Study the drawing (mm; zero at the part's minimum x, y, z) and answer. Coordinates: 2 decimals unless noted, no trailing zeros. Loops run counter-clockwise (first coordinate to the right, second up) from the corner with the lowest first, then second, coordinate; pieces in that order, holes last. Notation, with made-up numbers: (-25.75, 39.25) -> (19.25, 39.25) arc R35 ccw to (19.25, 75.25) -> close; hole circle Ø5 at (64.25, 20.5). An arc over 180 degrees is marked (long way). Answer as a JSON object with one key per item and string values. Group by question number.
Q1. Determine the mould class of the marked faces 1, 2 and 3 for opening direction Y: released by +Y, released by -Y, zero draft, split by the parting line, or undercut.
Q2. Straight lines are drawn through the part: line 1 along Y through (x, z) = (3, 50); line 2 along Y through (x, z) = (7.25, 50); line 3 along Y through (x, z) = (1, 49). For each, find the intervals that lie inside material, in ascending order. Write a range as [from, to].
Q3. The part is cut by section A-A on z = 50. Write down the section's boundary in (x, y), and give its area (3 significant figures).
Q4. Each of these flat-tipped pins is pushed along its axis until it touches: P1, Ø3, axis at x = 4, y = 142.5, coming from the +Z side; P2, Ø1.8, axis at y = 36, z = 49, coming from the -X side; P3, Ø5, axis at x = 7, y = 33.5, coming from the +Z side; P4, Ø9, axis at y = 180, z = 50, coming from the -X side. Where does it stop, or does it pass through?
Q5. The part is cut by section C-C on z = 78. Write down the section's boundary in (x, y), and give its area (3 significant figures).
Q6. The part is cut by section D-D on y = 35.5. Write down the section's boundary in (x, z), and give its area (3 significant figures).
Q7. The part is cut by section B-B on x = 7. Write down the section's boundary in (y, z).
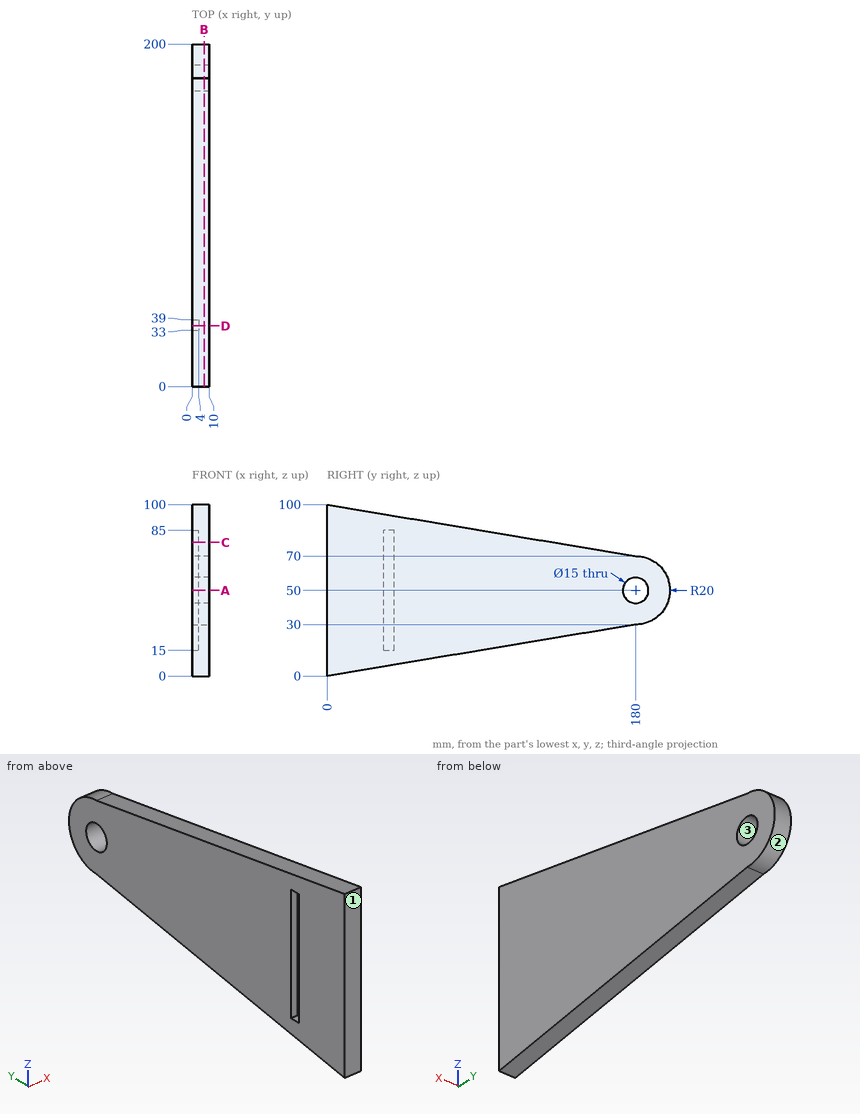
Final values:
{
 "1": {"face 1": "released by -Y", "face 2": "released by +Y", "face 3": "undercut"},
 "2": {"line 1": "y = [0, 33], [39, 172.5], [187.5, 200]", "line 2": "y = [0, 172.5], [187.5, 200]", "line 3": "y = [0, 33], [39, 172.57], [187.43, 199.97]"},
 "3": {"outline": "(0, 0) -> (10, 0) -> (10, 172.5) -> (0, 172.5) -> (0, 39) -> (4, 39) -> (4, 33) -> (0, 33) -> close; (0, 187.5) -> (10, 187.5) -> (10, 200) -> (0, 200) -> close", "area": "1,830 mm2"},
 "4": {"P1": "stops at z = 76.5", "P2": "stops at x = 4", "P3": "stops at z = 94.83", "P4": "passes through"},
 "5": {"outline": "(0, 0) -> (10, 0) -> (10, 132) -> (0, 132) -> (0, 39) -> (4, 39) -> (4, 33) -> (0, 33) -> close", "area": "1,300 mm2"},
 "6": {"outline": "(0, 5.92) -> (10, 5.92) -> (10, 94.08) -> (0, 94.08) -> (0, 85) -> (4, 85) -> (4, 15) -> (0, 15) -> close", "area": "602 mm2"},
 "7": {"outline": "(0, 0) -> (180, 30) arc R20 ccw to (180, 70) -> (0, 100) -> close; hole circle Ø15 at (180, 50)"}
}
